Can you work these out from the drawing? Everything is in mm from the part's minimum corner. A direction names the side the tool comes from. Coordinates: 2 decimals unless noted, no trailing zeros. Write each loop counter-clockwise with the first axis right and the second up, starting at its lowest first coordinate (ties: lowest second). Pieces come first, ordered by that corner, then holes. Notation, with made-up numbers: M 9,3.5 L 17,3.5 A20 cw 17,12.5 Z; hole C 65.5,-16 d6. An arc over 180 degrees is marked long. Write each question's results on one line, items separated by ' | '. Start each with the question number.
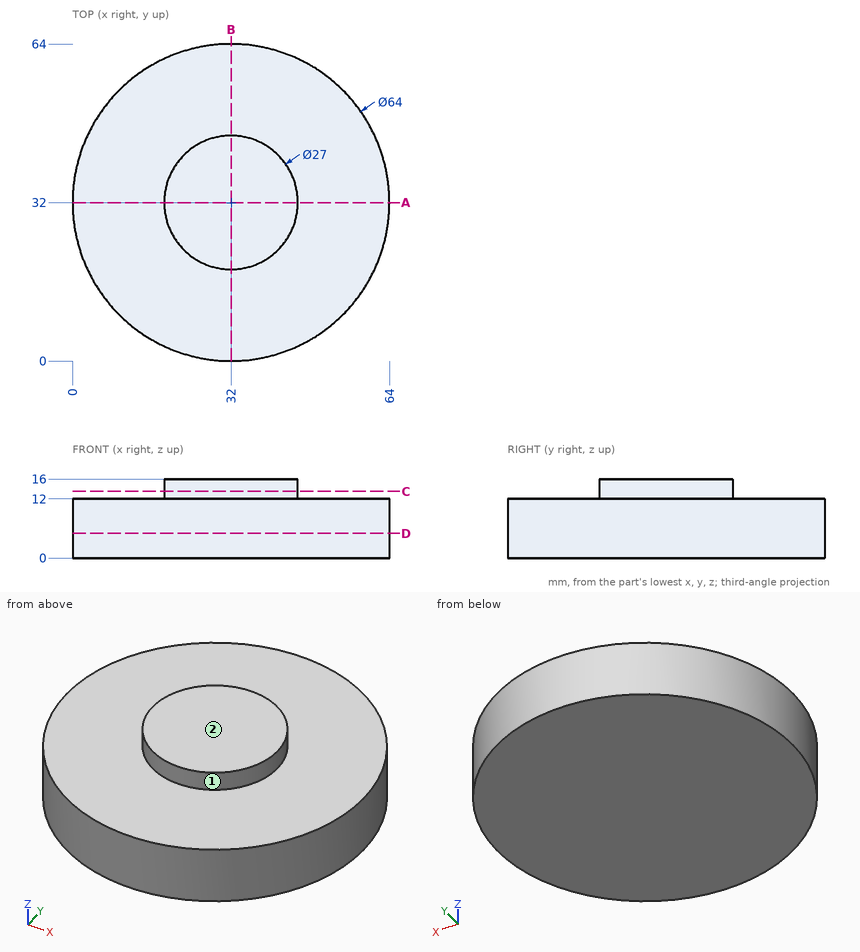
1) For the marked faces 1 and 2, which set-ups out of +Z, -Z, +X, -X, +Y, -Y let a thin tool reach every point of the face, with its end or its side?
2) I want a section at C-C, the plane z = 13.5. Write out the boundary of the cut face in (x, y).
3) I want a section at A-A, the plane y = 32. Write out the boundary of the cut face in (x, z).
4) Please list where these lines run through material, in increasing order: line 1 (Z direction, x = 20, y = 20); line 2 (X direction, y = 5, z = 6.25); line 3 (Y direction, x = 16, z = 2.5). Write a range as [from, to].
5) For pin 1 Ø2 at (y, z) = (23, 14) entering from +X; pin 2 Ø1 at (x, y) = (51, 41.5) entering from +Z; pin 3 Ø6 at (x, z) = (6.5, 11.5) entering from +Y, each with a flat end and sliding along its axis, tell me the tip position at first contact or that it passes through.
6) I want a section at D-D, the plane z = 5. Write out the boundary of the cut face in (x, y), then the cut area to 3 significant figures.
Output:
1) face 1: +Z | face 2: +Z, +X, -X, +Y, -Y
2) outline: C 32,32 d27
3) outline: M 0,0 L 64,0 L 64,12 L 45.5,12 L 45.5,16 L 18.5,16 L 18.5,12 L 0,12 Z
4) line 1: z = [0, 12] | line 2: x = [14.82, 49.18] | line 3: y = [4.29, 59.71]
5) pin 1: stops at x = 42.87 | pin 2: stops at z = 12 | pin 3: stops at y = 54.75
6) outline: C 32,32 d64 | area: 3,220 mm2
